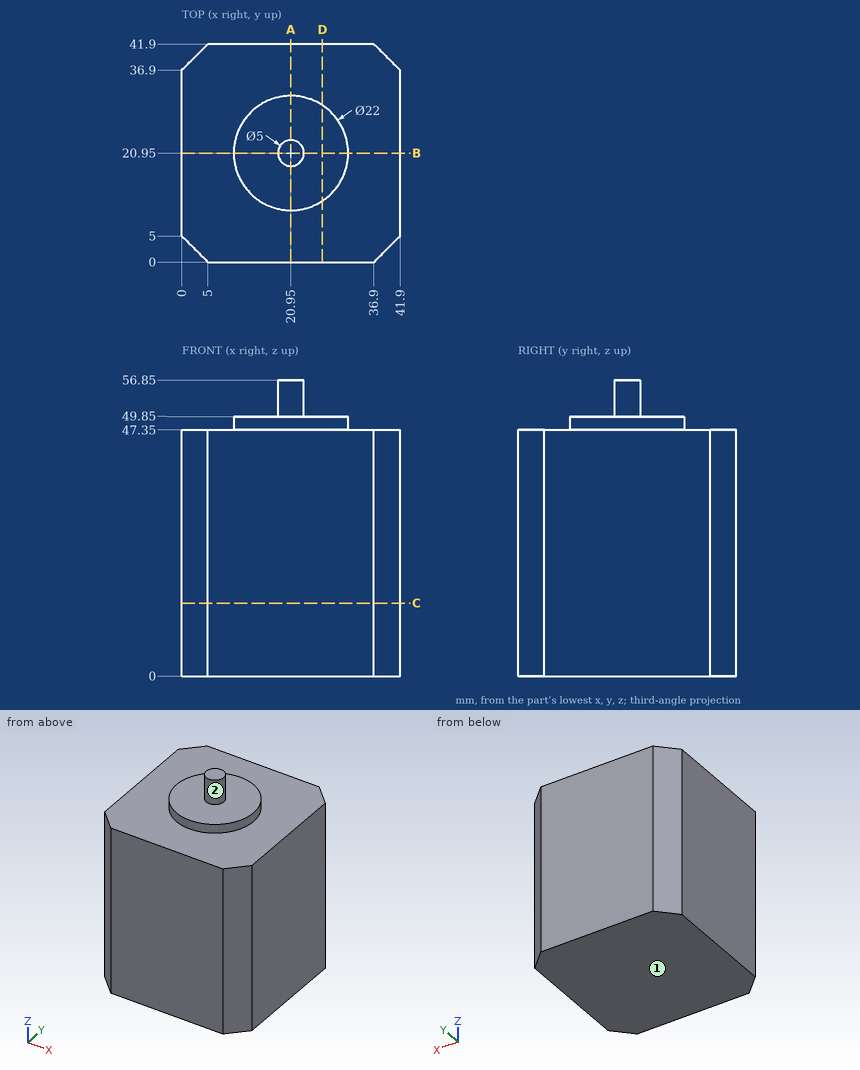
Here's the drawing with two shaded views (mm, measured from the low corner). I have some questions. A direction names the side the tool comes from. Give positions to 0.01 mm unless a question says otherwise; leave off trailing zeros. Loops run counter-clockwise (first coordinate to the right, second up) from the corner with the lowest first, then second, coordinate; pieces in that order, holes last. Notation, with made-up numbers: (40.25, -11.75) - (74.25, -11.75) arc R24 ccw to (74.25, 11.25) - close; hole circle Ø7 at (83, 21). An arc over 180 degrees is marked (long way). One line per item, written item: value.
(1) If we section it at D-D, the plane x = 27: List the corners of the cut face in (y, z) for me.
Verdict:
outline: (0, 0) - (41.9, 0) - (41.9, 47.35) - (30.14, 47.35) - (30.14, 49.85) - (11.76, 49.85) - (11.76, 47.35) - (0, 47.35) - close
(2) If we section it at C-C, the plane z = 14: List the corners of the cut face in (x, y) for me.
Verdict:
outline: (0, 5) - (5, 0) - (36.9, 0) - (41.9, 5) - (41.9, 36.9) - (36.9, 41.9) - (5, 41.9) - (0, 36.9) - close
(3) I need wall thicknesses on line 1 along Z through (x, y) = (23, 39.5); line 2 along Y through (x, z) = (3.5, 9.5); line 3 along Y through (x, z) = (29.5, 49). Which ranges of each line are inside material? Lowest first, please.
Verdict:
line 1: 0 to 47.35
line 2: 1.5 to 40.4
line 3: 14.03 to 27.87
(4) I'm going to push flat-ended pins straight in: pin 1 (1.5 mm diameter, centred on y = 9, z = 50.5, fed in from -X); pin 2 (6 mm diameter, centred on x = 15.5, y = 35.5, fed in from +Z). Where does each tip first touch, or does it pass through?
Verdict:
pin 1: through
pin 2: z = 47.35
(5) On a 3-axis mill with a long thin cutter (end or side, diameter ignored), from which of +Z, -Z, +X, -X, +Y, -Y can I reach the whole of each face in a straight line? I mean the marked faces 1 and 2. Say none if no direction works.
Verdict:
face 1: -Z, +X, -X, +Y, -Y
face 2: +Z
(6) If we section it at A-A, the plane x = 20.95: List the corners of the cut face in (y, z) for me.
Verdict:
outline: (0, 0) - (41.9, 0) - (41.9, 47.35) - (31.95, 47.35) - (31.95, 49.85) - (23.45, 49.85) - (23.45, 56.85) - (18.45, 56.85) - (18.45, 49.85) - (9.95, 49.85) - (9.95, 47.35) - (0, 47.35) - close
